CAD build for the part. Positions are in the model's coordinates, mm. Round coordinates to 2 decimals unless told otherwise and drop trailing zeros.
from build123d import *

# Parameters (mm, degrees)
SKETCH_1_R      = 22
SKETCH_1_R_2    = 9.5
SKETCH_1_R_3    = 1.3
SKETCH_1_R_4    = 1.5
SKETCH_1_R_5    = 1.035150144
EXTRUDE_1_DEPTH = 3


with BuildPart() as part:
    # 草图1 → 凸台-拉伸1 (new body)
    with BuildSketch(Plane.XY):
        Circle(SKETCH_1_R)
        Circle(SKETCH_1_R_2, mode=Mode.SUBTRACT)
        with Locations((8.264326198, -12.518023506)):
            Circle(SKETCH_1_R_3, mode=Mode.SUBTRACT)
        with Locations((-9.351530584, -11.728123283)):
            Circle(SKETCH_1_R_3, mode=Mode.SUBTRACT)
        with Locations((-14.043889946, 5.269644693)):
            Circle(SKETCH_1_R_3, mode=Mode.SUBTRACT)
        with Locations((0.671929263, 14.984942812)):
            Circle(SKETCH_1_R_3, mode=Mode.SUBTRACT)
        with Locations((14.459165069, 3.991559284)):
            Circle(SKETCH_1_R_3, mode=Mode.SUBTRACT)
        with Locations((6.708763262, 13.416128186)):
            Circle(SKETCH_1_R_4, mode=Mode.SUBTRACT)
        with Locations((14.832617994, -2.234601409)):
            Circle(SKETCH_1_R_4, mode=Mode.SUBTRACT)
        with Locations((2.4582988, -14.797187807)):
            Circle(SKETCH_1_R_4, mode=Mode.SUBTRACT)
        with Locations((-13.313305781, -6.910563594)):
            Circle(SKETCH_1_R_4, mode=Mode.SUBTRACT)
        with Locations((-10.686374275, 10.526224625)):
            Circle(SKETCH_1_R_4, mode=Mode.SUBTRACT)
        with Locations((-15.140028741, 9.670334022)):
            Circle(SKETCH_1_R_5, mode=Mode.SUBTRACT)
        with Locations((4.51850801, 17.387320545)):
            Circle(SKETCH_1_R_5, mode=Mode.SUBTRACT)
        with Locations((17.932620269, 1.075621048)):
            Circle(SKETCH_1_R_5, mode=Mode.SUBTRACT)
        with Locations((6.564460824, -16.722550178)):
            Circle(SKETCH_1_R_5, mode=Mode.SUBTRACT)
        with Locations((-13.875560362, -11.410725437)):
            Circle(SKETCH_1_R_5, mode=Mode.SUBTRACT)
        with BuildLine():
            ThreePointArc((-5.923480438, 11.007378412), (-6.772768209, 10.961109563), (-7.350473407, 11.585358894))
            ThreePointArc((-7.350473407, 11.585358894), (-8.407095271, 13.182328392), (-10.145967922, 13.984253106))
            ThreePointArc((-10.145967922, 13.984253106), (-10.968173498, 14.757231005), (-10.546653113, 15.804053534))
            ThreePointArc((-10.546653113, 15.804053534), (-6.942710719, 17.686117943), (-3.020854346, 18.758316529))
            ThreePointArc((-3.020854346, 18.758316529), (-1.999770978, 18.277790153), (-2.076575062, 17.151904734))
            ThreePointArc((-2.076575062, 17.151904734), (-2.805565056, 15.381217034), (-2.49364552, 13.491913579))
            ThreePointArc((-2.49364552, 13.491913579), (-2.492417598, 12.641367275), (-3.146384684, 12.097531295))
            ThreePointArc((-3.146384684, 12.097531295), (-4.567572841, 11.63560391), (-5.923480438, 11.007378412))
        make_face(mode=Mode.SUBTRACT)
        with BuildLine():
            ThreePointArc((10.533149631, 6.730732416), (9.654659288, 7.939619262), (8.638182844, 9.035031663))
            ThreePointArc((8.638182844, 9.035031663), (8.3317342, 9.82845447), (8.74690987, 10.570788416))
            ThreePointArc((8.74690987, 10.570788416), (9.939204005, 12.069186239), (10.164538529, 13.97076077))
            ThreePointArc((10.164538529, 13.97076077), (10.645608702, 14.991588048), (11.771453052, 14.91418429))
            ThreePointArc((11.771453052, 14.91418429), (14.675082118, 12.068221279), (16.90672384, 8.669641804))
            ThreePointArc((16.90672384, 8.669641804), (16.765248211, 7.550042997), (15.67073378, 7.275170293))
            ThreePointArc((15.67073378, 7.275170293), (13.761439408, 7.421308386), (12.060993483, 6.540828404))
            ThreePointArc((12.060993483, 6.540828404), (11.252455327, 6.276827318), (10.533149631, 6.730732416))
        make_face(mode=Mode.SUBTRACT)
        with BuildLine():
            ThreePointArc((9.656229164, -7.937709892), (10.534480431, -6.728649348), (11.262171037, -5.423421755))
            ThreePointArc((11.262171037, -5.423421755), (11.92206313, -4.886790644), (12.756361003, -5.052252365))
            ThreePointArc((12.756361003, -5.052252365), (14.549861167, -5.72316108), (16.427998213, -5.349848101))
            ThreePointArc((16.427998213, -5.349848101), (17.547521507, -5.491920046), (17.821811196, -6.586580728))
            ThreePointArc((17.821811196, -6.586580728), (16.012410255, -10.227547009), (13.469784317, -13.400183224))
            ThreePointArc((13.469784317, -13.400183224), (12.361264202, -13.611606964), (11.761621167, -12.655602219))
            ThreePointArc((11.761621167, -12.655602219), (11.310602344, -10.794596211), (9.947749431, -9.449459311))
            ThreePointArc((9.947749431, -9.449459311), (9.446817447, -8.762074651), (9.656229164, -7.937709892))
        make_face(mode=Mode.SUBTRACT)
        with BuildLine():
            ThreePointArc((-4.565271804, -11.636506922), (-3.143992328, -12.098153257), (-1.677778356, -12.386890642))
            ThreePointArc((-1.677778356, -12.386890642), (-0.96349397, -12.848657184), (-0.863045197, -13.693252097))
            ThreePointArc((-0.863045197, -13.693252097), (-0.946895272, -15.60629431), (-0.011477266, -17.277148731))
            ThreePointArc((-0.011477266, -17.277148731), (0.199356008, -18.3857813), (-0.756967992, -18.98491505))
            ThreePointArc((-0.756967992, -18.98491505), (-4.778868338, -18.389192951), (-8.58193931, -16.951410492))
            ThreePointArc((-8.58193931, -16.951410492), (-9.12556679, -15.962478742), (-8.401652136, -15.096762613))
            ThreePointArc((-8.401652136, -15.096762613), (-6.771102726, -14.092735739), (-5.912946223, -12.380915433))
            ThreePointArc((-5.912946223, -12.380915433), (-5.414001059, -11.692087264), (-4.565271804, -11.636506922))
        make_face(mode=Mode.SUBTRACT)
        with BuildLine():
            ThreePointArc((-12.477722307, 0.745953104), (-12.47757455, -0.748420566), (-12.299095087, -2.232097677))
            ThreePointArc((-12.299095087, -2.232097677), (-12.517535151, -3.054116206), (-13.289752269, -3.410642848))
            ThreePointArc((-13.289752269, -3.410642848), (-15.135074629, -3.922059242), (-16.435091554, -5.328017043))
            ThreePointArc((-16.435091554, -5.328017043), (-17.424312718, -5.871117707), (-18.289643143, -5.146742046))
            ThreePointArc((-18.289643143, -5.146742046), (-18.965913316, -1.137599261), (-18.773714501, 2.923635383))
            ThreePointArc((-18.773714501, 2.923635383), (-18.001174645, 3.746252557), (-16.954127749, 3.325289805))
            ThreePointArc((-16.954127749, 3.325289805), (-15.49537397, 2.084806529), (-13.60215117, 1.797632761))
            ThreePointArc((-13.60215117, 1.797632761), (-12.792854116, 1.535967322), (-12.477722307, 0.745953104))
        make_face(mode=Mode.SUBTRACT)
    extrude(amount=EXTRUDE_1_DEPTH)


solid = part.part
Item 1: Wall check: L1, parallel to X at y = -16, z = 1.85; L2, parallel to Y at x = 16.5, z = 2.1; L3, parallel to Y at x = -14.5, z = 0.25. Give the ranges that are in metal, low to high.
Verdict:
L1: x = -15.1 to -9.13, -0.83 to 1.56, 3.35 to 5.82, 7.31 to 15.1
L2: y = -14.55 to -9.42, -5.32 to 7.34, 9.42 to 14.55
L3: y = -16.55 to -12.24, -10.59 to -7.83, -5.99 to -3.62, 1.8 to 4.05, 6.49 to 8.86, 10.48 to 16.55
Item 2: Flat gauge pins, fed straight in: P1, Ø2.5, axis at x = 6.56, y = -16.72, coming from the -Z side; P2, Ø1.5, axis at y = -16.5, z = 1, coming from the -X side. Where does each tip first touch, or does it go through?
Verdict:
P1: stops at z = 0
P2: stops at x = -15.36
Item 3: Cut at A-A (z = 1.8). State how many separate pieces and enclosed holes the cut face has, plus the area to 3 significant figures.
Verdict:
separate pieces: 1
enclosed holes: 21
area: 936 mm2
